Here's how the part is built. I have some questions about the finished solid (model axes, mm). Face numbers are marked on the shaded views. A direction names the side the tool comes from. Round coordinates to 2 decimals unless told otherwise and drop trailing zeros. Loops run counter-clockwise (first coordinate to the right, second up) from the corner with the lowest first, then second, coordinate; pieces in that order, holes last. Notation, with made-up numbers: M 20,-5.75 L 27,-5.75 A24 ccw 27,31.25 Z; hole C 50.5,28.25 d11. An arc over 180 degrees is marked long. Use a Markdown table: item, result.
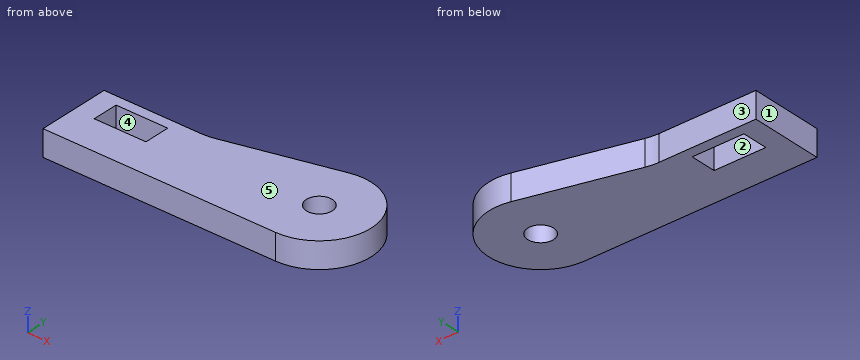
from build123d import *

# Parameters (mm, degrees)
SKETCH1_R           = 2.5
SKETCH1_W           = 10
SKETCH1_H           = 5
BOSS_EXTRUDE1_DEPTH = 5


with BuildPart() as part:
    # Sketch1 → Boss-Extrude1 (new body)
    with BuildSketch(Plane.XY):
        with BuildLine():
            Line((-24.313432836, 0), (20.686567164, 0))
            ThreePointArc((20.686567164, 0), (30.610164404, 11.23378192), (18.237856194, 19.695556435))
            Line((18.237856194, 19.695556435), (-3.108002795, 14.304443565))
            ThreePointArc((-3.108002795, 14.304443565), (-4.322931845, 14.07640276), (-5.556713765, 14))
            Line((-5.556713765, 14), (-24.313432836, 14))
            Line((-24.313432836, 14), (-24.313432836, 0))
        make_face()
        with Locations((20.686567164, 10)):
            Circle(SKETCH1_R, mode=Mode.SUBTRACT)
        with Locations((-15.313432836, 9.5)):
            Rectangle(SKETCH1_W, SKETCH1_H, mode=Mode.SUBTRACT)
    extrude(amount=BOSS_EXTRUDE1_DEPTH)


solid = part.part
1. Which directions (+Z, -Z, +X, -X, +Y, -Y) give clear straight access to the entire face, cutting with the end or side of a thin tool? Please do the marked faces 4 and 5.
Answer sheet:
| item | result |
|---|---|
| face 4 | +Z, -Z |
| face 5 | +Z, +X, -X, +Y, -Y |
2. We'd pull the mould along X, two halves only. Please class the marked faces 1, 2 and 3: +X half, -X half, draft (parallel to the pull), parting line (faces both ways), or undercut.
Answer sheet:
| item | result |
|---|---|
| face 1 | -X half |
| face 2 | undercut |
| face 3 | draft |
3. Imagine slicing it at D-D, the plane y = 1.5. Write out the boundary of the cut face in (x, z).
Answer sheet:
| item | result |
|---|---|
| outline | M -24.31,0 L 25.95,0 L 25.95,5 L -24.31,5 Z |
4. Imagine slicing it at B-B, the plane y = 10. Write out the boundary of the cut face in (x, z), then the cut area to 3 significant figures.
Answer sheet:
| item | result |
|---|---|
| outline | M -24.31,0 L -20.31,0 L -20.31,5 L -24.31,5 Z; M -10.31,0 L 18.19,0 L 18.19,5 L -10.31,5 Z; M 23.19,0 L 30.69,0 L 30.69,5 L 23.19,5 Z |
| area | 200 mm2 |
5. For pin 1 Ø1 at (x, z) = (-11, 1) entering from +Y; pin 2 Ø1.5 at (y, z) = (17.5, 1) entering from +X, each with a flat end and sliding along its axis, tell me the tip position at first contact or that it passes through.
Answer sheet:
| item | result |
|---|---|
| pin 1 | y = 14 |
| pin 2 | x = 28.06 |
6. Imagine slicing it at A-A, the plane x = -18. Write out the boundary of the cut face in (y, z), then the cut area to 3 significant figures.
Answer sheet:
| item | result |
|---|---|
| outline | M 0,0 L 7,0 L 7,5 L 0,5 Z; M 12,0 L 14,0 L 14,5 L 12,5 Z |
| area | 45.0 mm2 |
7. I need wall thicknesses on probe 1 along X at (y, z) = (11.5, 4.35); probe 2 along Y at (x, z) = (-7, 2.1); probe 3 along Y at (x, z) = (19.5, 2.4). Which ranges of each line are inside material? Lowest first, please. Write a range as from..to.
Answer sheet:
| item | result |
|---|---|
| probe 1 | -24.31..-20.31, -10.31..18.69, 22.69..30.57 |
| probe 2 | 0..14 |
| probe 3 | 0..7.8, 12.2..19.93 |
8. Imagine slicing it at C-C, the plane z = 1.8. Write out the boundary of the cut face in (x, y), then the cut area to 3 significant figures.
Answer sheet:
| item | result |
|---|---|
| outline | M -24.31,0 L 20.69,0 A10 ccw long 18.24,19.7 L -3.11,14.3 A10 cw -5.56,14 L -24.31,14 Z; hole M -20.31,7 L -10.31,7 L -10.31,12 L -20.31,12 Z; hole C 20.69,10 d5 |
| area | 796 mm2 |
